from build123d import *

# Parameters (mm, degrees)
BOSS_EXTRUDE1_DEPTH = 0.08
BOSS_EXTRUDE2_DEPTH = 10
SKETCH1_4_W         = 175.5
SKETCH1_4_H         = 2
BOSS_EXTRUDE3_DEPTH = 15.46


with BuildPart() as part:
    # Sketch1 → Boss-Extrude1 (new body)
    with BuildSketch(Plane(origin=(0, 0, 0), x_dir=(1, 0, 0), z_dir=(0, 1, 0))):
        Polygon((-115, 0), (-111, -6.92820323), (111, -6.92820323), (115, 0), (4, 192.25763964), (-4, 192.25763964), align=None)
    extrude(amount=BOSS_EXTRUDE1_DEPTH)

    # Sketch1<3> → Boss-Extrude2 (add)
    with BuildSketch(Plane(origin=(0, 0, 0), x_dir=(1, 0, 0), z_dir=(0, 1, 0))):
        Polygon((-103.375, 20.135090638), (-115, 0), (-111, -6.92820323), (-87.75, -6.92820323), (-87.75, -4.92820323), (-109.845299462, -4.92820323), (-112.690598923, 0), (-101.642949192, 19.135090638), align=None)
        Polygon((-4, 192.25763964), (-15.625, 172.122549002), (-13.892949192, 171.122549002), (-2.845299462, 190.25763964), (2.845299462, 190.25763964), (13.892949192, 171.122549002), (15.625, 172.122549002), (4, 192.25763964), align=None)
        Polygon((87.75, -4.92820323), (87.75, -6.92820323), (111, -6.92820323), (115, 0), (103.375, 20.135090638), (101.642949192, 19.135090638), (112.690598923, 0), (109.845299462, -4.92820323), align=None)
    extrude(amount=BOSS_EXTRUDE2_DEPTH)

    # Sketch1<4> → Boss-Extrude3 (add)
    with BuildSketch(Plane(origin=(0, 0, 0), x_dir=(1, 0, 0), z_dir=(0, 1, 0))):
        Polygon((-15.625, 172.122549002), (-103.375, 20.135090638), (-101.642949192, 19.135090638), (-13.892949192, 171.122549002), align=None)
        with Locations((0, -5.92820323)):
            Rectangle(SKETCH1_4_W, SKETCH1_4_H)
        Polygon((103.375, 20.135090638), (15.625, 172.122549002), (13.892949192, 171.122549002), (101.642949192, 19.135090638), align=None)
    extrude(amount=BOSS_EXTRUDE3_DEPTH)


solid = part.part
Can you work these out from the model? Positions are in its coordinate system, mm. A direction names the side the tool comes from. Round coordinates to 2 decimals unless told otherwise and drop trailing zeros. Loops run counter-clockwise (first coordinate to the right, second up) from the corner with the lowest first, then second, coordinate; pieces in that order, holes last. Notation, with made-up numbers: (58, -40) - (76, -40) arc R13 cw to (76, -25) - close; hole circle Ø2 at (81, 49). An arc over 180 degrees is marked (long way). Write item = value, one per line. Start each with the question number.
(1) If we section it at B-B (z = -157): Please give me the cut outline in (x, y).
(2) If I drill on probe 1 along Z at (x, y) = (-44.5, 7); probe 2 along X at (y, z) = (13.25, -94); probe 3 along Z at (x, y) = (49.5, 5.5), over which ranges is the centre line in solid material (lowest first)? Write a range as [from, to].
(3) For faces 5 (the face through (111.288, 4.971, 2.43)), 6 (the face through (-110, 10, -6)), 7 (the face through (-113.028, 4.93, 3.416)), which set-ups out of +Z, -Z, +X, -X, +Y, -Y let a thin tool reach every point of the face, with its end or its side?
(4) If we section it at C-C (x = -38): Please give me the cut outline in (y, z).
(5) If we mould it in two halves opening along Z, with no side actions, what happens to faces 1 (the face through (2, 8, 4.928)), 2 (the face through (-111.248, 4.971, 2.499)), 3 (the face through (-58.723, 7.622, -97.475)), 4 (the face through (110, 10, -5))? For each: released by +Z, released by -Z, zero draft, split by the parting line, or undercut.
(6) For P1, Ø3, axis at x = -10, z = -85.5, coming from the +Y side; P2, Ø1, axis at y = 11.5, z = 5.5, coming from the -X side; P3, Ø10.5, axis at x = -2, z = -184.5, coming from the +Y side, each with a flat end and sliding along its axis, tell me the tip position at first contact or that it passes through.
(7) If we section it at A-A (y = 6.5): Please give me the cut outline in (x, z).
Ans:
q1.outline = (-24.36, 0) - (24.36, 0) - (24.36, 15.46) - (22.05, 15.46) - (22.05, 0.08) - (-22.05, 0.08) - (-22.05, 15.46) - (-24.36, 15.46) - close
q2.probe_1 = [-122.11, -118.11], [4.93, 6.93]
q2.probe_2 = [-60.73, -58.42], [58.42, 60.73]
q2.probe_3 = [-113.45, -109.45], [4.93, 6.93]
q3.face_5 = +Y
q3.face_6 = +Z, -X, +Y
q3.face_7 = +Z, -X, +Y, -Y
q4.outline = (0, -133.37) - (15.46, -133.37) - (15.46, -129.37) - (0.08, -129.37) - (0.08, 4.93) - (15.46, 4.93) - (15.46, 6.93) - (0, 6.93) - close
q5.face_1 = undercut
q5.face_2 = undercut
q5.face_3 = released by -Z
q5.face_4 = zero draft
q6.P1 = 0.08
q6.P2 = -87.75
q6.P3 = 10
q7.outline = (-115, 0) - (-4, -192.26) - (4, -192.26) - (115, 0) - (111, 6.93) - (-111, 6.93) - close; hole (-112.69, 0) - (-2.85, -190.26) - (2.85, -190.26) - (112.69, 0) - (109.85, 4.93) - (-109.85, 4.93) - close
